```python
from build123d import *

# Parameters (mm, degrees)
F0_R     = 11.05
F0_R_2   = 13.55
F1_DEPTH = 7


with BuildPart() as f1:
    # F0 (on Top) → F1 (new body)
    with BuildSketch(Plane.XY):
        with BuildLine():
            ThreePointArc((2.6065338711, -13.2969350295), (10.4623380263, -8.6105739079), (13.55, 0))
            ThreePointArc((13.55, 0), (13.0425271945, 3.6735520114), (11.5581203867, 7.0719412559))
            ThreePointArc((11.5581203867, 7.0719412559), (-1.2547280417, 13.4917811108), (-12.6639989198, 4.8192978077))
            ThreePointArc((-12.6639989198, 4.8192978077), (-10.3603872444, -8.7329763624), (2.6065338711, -13.2969350295))
        make_face()
        Circle(F0_R, mode=Mode.SUBTRACT)
        with BuildLine():
            ThreePointArc((11.5581203867, 7.0719412559), (13.0425271945, 3.6735520114), (13.55, 0))
            ThreePointArc((13.55, 0), (10.4623380263, -8.6105739079), (2.6065338711, -13.2969350295))
            Line((2.6065338711, -13.2969350295), (12.3875978298, -24.2038302976))
            Line((12.3875978298, -24.2038302976), (-14.9941514566, -23.8444135863))
            ThreePointArc((-14.9941514566, -23.8444135863), (-18.3532690256, -26.2108119603), (-22.267239092, -27.461551912))
            Line((-22.267239092, -27.461551912), (49.0895092572, -28.3981906763))
            Line((49.0895092572, -28.3981906763), (13.0464962981, 31.8175852156))
            ThreePointArc((13.0464962981, 31.8175852156), (13.4235339021, 30.0051079331), (13.55, 28.1581543386))
            ThreePointArc((13.55, 28.1581543386), (13.2562145915, 25.351862354), (12.3875978298, 22.6672600574))
            Line((12.3875978298, 22.6672600574), (28.0773907901, 0))
            Line((28.0773907901, 0), (11.5581203867, 7.0719412559))
        make_face()
        with Locations((24.3843801233, -14.0799748264)):
            Circle(F0_R_2, mode=Mode.SUBTRACT)
        with BuildLine():
            ThreePointArc((-12.6639989198, 4.8192978077), (-1.2547280417, 13.4917811108), (11.5581203867, 7.0719412559))
            Line((11.5581203867, 7.0719412559), (12.3875978298, 22.6672600574))
            ThreePointArc((12.3875978298, 22.6672600574), (0, 14.6081543386), (-12.3875978298, 22.6672600574))
            Line((-12.3875978298, 22.6672600574), (-12.6639989198, 4.8192978077))
        make_face()
        with BuildLine():
            Line((-14.9941514566, -23.8444135863), (2.6065338711, -13.2969350295))
            ThreePointArc((2.6065338711, -13.2969350295), (-10.3603872444, -8.7329763624), (-12.6639989198, 4.8192978077))
            Line((-12.6639989198, 4.8192978077), (-25.4531481717, 0))
            Line((-25.4531481717, 0), (-12.3875978298, 22.6672600574))
            ThreePointArc((-12.3875978298, 22.6672600574), (-13.4461101823, 26.4834540771), (-13.3560221409, 30.4427051857))
            Line((-13.3560221409, 30.4427051857), (-32.9787461707, -3.600513583))
            ThreePointArc((-32.9787461707, -3.600513583), (-18.5911674875, -1.8305608799), (-10.8371028035, -14.0784028862))
            ThreePointArc((-10.8371028035, -14.0784028862), (-11.9196052449, -19.3853798623), (-14.9941514566, -23.8444135863))
        make_face()
        with BuildLine():
            ThreePointArc((-12.3875978298, 22.6672600574), (0, 14.6081543386), (12.3875978298, 22.6672600574))
            ThreePointArc((12.3875978298, 22.6672600574), (13.2562145915, 25.351862354), (13.55, 28.1581543386))
            ThreePointArc((13.55, 28.1581543386), (13.4235339021, 30.0051079331), (13.0464962981, 31.8175852156))
            Line((13.0464962981, 31.8175852156), (9.3890984881, 37.9278692567))
            ThreePointArc((9.3890984881, 37.9278692567), (0.4816570964, 41.6995909847), (-8.6712487219, 38.5702600624))
            Line((-8.6712487219, 38.5702600624), (-13.3560221409, 30.4427051857))
            ThreePointArc((-13.3560221409, 30.4427051857), (-13.4461101823, 26.4834540771), (-12.3875978298, 22.6672600574))
        make_face()
        with Locations((0, 28.1581543386)):
            Circle(F0_R, mode=Mode.SUBTRACT)
        with BuildLine():
            ThreePointArc((-22.267239092, -27.461551912), (-18.3532690256, -26.2108119603), (-14.9941514566, -23.8444135863))
            ThreePointArc((-14.9941514566, -23.8444135863), (-11.9196052449, -19.3853798623), (-10.8371028035, -14.0784028862))
            ThreePointArc((-10.8371028035, -14.0784028862), (-18.5911674875, -1.8305608799), (-32.9787461707, -3.600513583))
            Line((-32.9787461707, -3.600513583), (-37.7601482446, -11.895708306))
            ThreePointArc((-37.7601482446, -11.895708306), (-35.4713085242, -21.872174986), (-26.8575138424, -27.4012993168))
            Line((-26.8575138424, -27.4012993168), (-22.267239092, -27.461551912))
        make_face()
        with Locations((-24.3871028035, -14.0784028862)):
            Circle(F0_R, mode=Mode.SUBTRACT)
        with BuildLine():
            Line((-46.5486845968, -27.1428302263), (-26.8575138424, -27.4012993168))
            ThreePointArc((-26.8575138424, -27.4012993168), (-35.4713085242, -21.872174986), (-37.7601482446, -11.895708306))
            Line((-37.7601482446, -11.895708306), (-46.5486845968, -27.1428302263))
        make_face()
        with BuildLine():
            Line((0, 53.6139011383), (-8.6712487219, 38.5702600624))
            ThreePointArc((-8.6712487219, 38.5702600624), (0.4816570964, 41.6995909847), (9.3890984881, 37.9278692567))
            Line((9.3890984881, 37.9278692567), (0, 53.6139011383))
        make_face()
        with Locations((24.3843801233, -14.0799748264)):
            Circle(F0_R_2)
        with Locations((24.3843801233, -14.0799748264)):
            Circle(F0_R, mode=Mode.SUBTRACT)
    extrude(amount=F1_DEPTH)


solid = f1.part
```
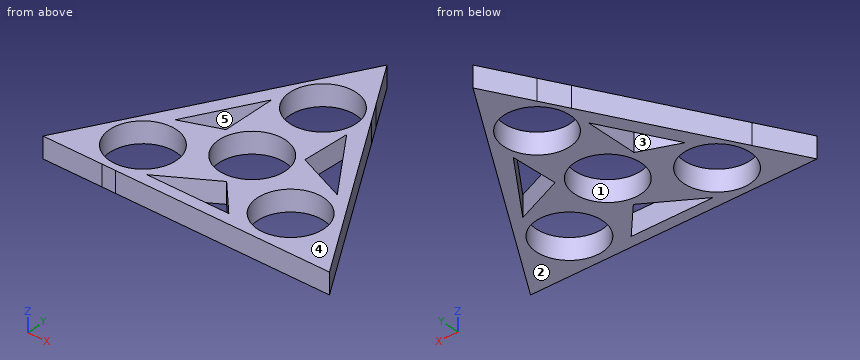
CAD build for the part. Positions are in the model's coordinates, mm. Face numbers are marked on the shaded views. A direction names the side the tool comes from. Round coordinates to 2 decimals unless told otherwise and drop trailing zeros. Loops run counter-clockwise (first coordinate to the right, second up) from the corner with the lowest first, then second, coordinate; pieces in that order, holes last. Notation, with made-up numbers: M -26.5,-38 L -0.5,-38 A13 ccw -0.5,-31 Z; hole C 26.25,51.5 d8. An arc over 180 degrees is marked long. Use a Markdown table: item, result. Add a question column.
(1) Cut at A-A (y = -17.5). Give the cut face in (x, z), and give its area (3 significant figures).
(2) Pull direction X, two halves, no side cores. Call the marked faces 1, 2 and 3: +X half, -X half, draft (parallel to the pull), parting line (faces both ways), or undercut.
(3) Cut at C-C (x = -16.5). Give the cut face in (y, z), and give its area (3 significant figures).
(4) Drill centre lines: line 1 (Y direction, x = -5, z = 3.75); line 2 (X direction, y = -7, z = 6); line 3 (Y direction, x = 27, z = 3.75). Where is each one in solid material? Low to high.
(5) Flat gauge pins, fed straight in: pin 1 (1.5 mm diameter, centred on y = -9, z = 2.5, fed in from +X); pin 2 (1 mm diameter, centred on y = -19, z = 1, fed in from -X); pin 3 (2 mm diameter, centred on y = -16, z = 1.5, fed in from +X). Where does each tip first touch, or does it go through?
(6) Cut at B-B (z = 3.5). Give the cut face in (x, y).
(7) Cut at D-D (y = 26). Give the cut face in (x, z).
(8) Which spindle directions (+Z, -Z, +X, -X, +Y, -Y) get a long thin tool onto all of the face, cutting with end or side? Do the marked faces 4 and 5. Say none if no direction does.
Geometry says:
| question | item | result |
|---|---|---|
| 1 | outline | M -40.99,0 L -34.89,0 L -34.89,7 L -40.99,7 Z; M -13.88,0 L -4.41,0 L -4.41,7 L -13.88,7 Z; M 6.38,0 L 13.88,0 L 13.88,7 L 6.38,7 Z; M 34.89,0 L 42.57,0 L 42.57,7 L 34.89,7 Z |
| 1 | area | 215 mm² |
| 2 | face 1 | undercut |
| 2 | face 2 | draft |
| 2 | face 3 | undercut |
| 3 | outline | M -27.54,0 L -21.82,0 L -21.82,7 L -27.54,7 Z; M -6.34,0 L 3.37,0 L 3.37,7 L -6.34,7 Z; M 15.53,0 L 24.99,0 L 24.99,7 L 15.53,7 Z |
| 3 | area | 174 mm² |
| 4 | line 1 | y = -27.69 to -23.98, -17.86 to -9.85, 9.85 to 18.3, 38.01 to 44.94 |
| 4 | line 2 | x = -34.94 to -32.87, -15.9 to -8.55, 8.55 to 15.9, 32.87 to 36.28 |
| 4 | line 3 | y = -28.11 to -24.82, -3.34 to 0.46, 1.56 to 8.51 |
| 5 | pin 1 | stops at x = 37.93 |
| 5 | pin 2 | stops at x = -42.14 |
| 5 | pin 3 | stops at x = 42.27 |
| 6 | outline | M -46.55,-27.14 L 49.09,-28.4 L 0,53.61 Z; hole C -24.39,-14.08 d22.1; hole M -25.45,0 L -12.66,4.82 L -12.39,22.67 Z; hole M -14.99,-23.84 L 12.39,-24.2 L 2.61,-13.3 Z; hole C 0,0 d22.1; hole C 0,28.16 d22.1; hole M 11.56,7.07 L 28.08,0 L 12.39,22.67 Z; hole C 24.38,-14.08 d22.1 |
| 7 | outline | M -15.92,0 L -10.84,0 L -10.84,7 L -15.92,7 Z; M 10.84,0 L 16.53,0 L 16.53,7 L 10.84,7 Z |
| 8 | face 4 | +Z, +X, -X, +Y, -Y |
| 8 | face 5 | +Z, -Z |
